```python
from build123d import *

# Parameters (mm, degrees)
SKETCH1_W           = 127
SKETCH1_H           = 127
BOSS_EXTRUDE1_DEPTH = 127
SKETCH2_W           = 96.52
SKETCH2_H           = 96.52
CUT_EXTRUDE1_DEPTH  = 118.11
SKETCH3_W           = 101.6
SKETCH3_H           = 101.6
SKETCH3_W_2         = 96.52
SKETCH3_H_2         = 96.52
CUT_EXTRUDE2_DEPTH  = 6.35
SKETCH5_W           = 96.52
SKETCH5_H           = 105.41
CUT_EXTRUDE3_DEPTH  = 6.35
SKETCH6_W           = 109.22
SKETCH6_H           = 105.41
CUT_EXTRUDE4_DEPTH  = 6.35
CHAMFER1_SIZE       = 1.016
FILLET2_R           = 0.762
FILLET3_R           = 0.762
FILLET4_R           = 0.762


with BuildPart() as part:
    # Sketch1 → Boss-Extrude1 (new body)
    with BuildSketch(Plane.XY):
        Rectangle(SKETCH1_W, SKETCH1_H)
    extrude(amount=BOSS_EXTRUDE1_DEPTH)

    # Sketch2 → Cut-Extrude1 (cut)
    with BuildSketch(Plane(origin=(0, 63.5, 0), x_dir=(1, 0, 0), z_dir=(0, 1, 0))):
        with Locations((0, -63.5)):
            Rectangle(SKETCH2_W, SKETCH2_H)
    extrude(amount=-CUT_EXTRUDE1_DEPTH, mode=Mode.SUBTRACT)

    # Sketch3 → Cut-Extrude2 (cut)
    with BuildSketch(Plane(origin=(0, 63.5, 0), x_dir=(1, 0, 0), z_dir=(0, 1, 0))):
        with Locations((0, -63.5)):
            Rectangle(SKETCH3_W, SKETCH3_H)
        with Locations((0, -63.5)):
            Rectangle(SKETCH3_W_2, SKETCH3_H_2, mode=Mode.SUBTRACT)
    extrude(amount=-CUT_EXTRUDE2_DEPTH, mode=Mode.SUBTRACT)

    # Sketch5 → Cut-Extrude3 (cut)
    with BuildSketch(Plane.XY.offset(15.24)):
        with Locations((0, -1.905)):
            Rectangle(SKETCH5_W, SKETCH5_H)
    cut_extrude3 = extrude(amount=-CUT_EXTRUDE3_DEPTH, mode=Mode.SUBTRACT)

    # Mirror1: Cut-Extrude3 across plane
    add(cut_extrude3.mirror(Plane(origin=(0, 0, 63.5), x_dir=(1, 0, 0), z_dir=(0, 0, -1))), mode=Mode.SUBTRACT)

    # Sketch6 → Cut-Extrude4 (cut)
    with BuildSketch(Plane.ZY.offset(-48.26)):
        with Locations((63.5, -1.905)):
            Rectangle(SKETCH6_W, SKETCH6_H)
    cut_extrude4 = extrude(amount=-CUT_EXTRUDE4_DEPTH, mode=Mode.SUBTRACT)

    # Mirror2: Cut-Extrude4 across plane
    add(cut_extrude4.mirror(Plane(origin=(0, 0, 0), x_dir=(0, 0, 1), z_dir=(1, 0, 0))), mode=Mode.SUBTRACT)

    # Chamfer1
    chamfer1_edges = [part.edges().sort_by_distance(p)[0] for p in [
        (0, -63.5, 127),
        (0, -63.5, 0),
        (63.5, -63.5, 63.5),
        (-63.5, -63.5, 63.5),
    ]]
    chamfer(chamfer1_edges, length=CHAMFER1_SIZE)

    # Fillet2
    fillet2_edges = [part.edges().sort_by_distance(p)[0] for p in [
        (54.61, -1.905, 8.89),
        (54.61, -1.905, 118.11),
        (-54.61, -1.905, 8.89),
        (-54.61, -1.905, 118.11),
    ]]
    fillet(fillet2_edges, radius=FILLET2_R)

    # Fillet3
    fillet3_edges = [part.edges().sort_by_distance(p)[0] for p in [
        (-50.8, 60.325, 114.3),
        (-50.8, 60.325, 12.7),
        (50.8, 60.325, 12.7),
        (50.8, 60.325, 114.3),
        (-48.26, 53.975, 15.24),
        (48.26, 53.975, 15.24),
        (48.26, 53.975, 111.76),
        (-48.26, 53.975, 111.76),
    ]]
    fillet(fillet3_edges, radius=FILLET3_R)

    # Fillet4
    fillet4_edges = [part.edges().sort_by_distance(p)[0] for p in [
        (54.61, 50.8, 63.5),
        (-54.61, 50.8, 63.5),
        (0, 50.8, 8.89),
        (0, 50.8, 118.11),
        (-54.386815367, 50.8, 9.113184633),
        (54.386815367, 50.8, 9.113184633),
        (-54.386815367, 50.8, 117.886815367),
        (54.386815367, 50.8, 117.886815367),
    ]]
    fillet(fillet4_edges, radius=FILLET4_R)


solid = part.part
```
Check sheet for the modelled part. Datum: model origin and axes. Units: mm. A direction names the side the tool comes from. Give positions to 0.01 mm unless a question says otherwise; leave off trailing zeros. Write each loop counter-clockwise with the first axis right and the second up, starting at its lowest first coordinate (ties: lowest second). Pieces come first, ordered by that corner, then holes.
Item 1: Gauge pin test, flat end, axial feed: pin 1 (8 mm diameter, centred on x = -23.5, z = 41, fed in from +Y). Record the tip position at first contact, or that the pin passes through.
Item 2: Cross-section at B-B (z = 63.5). Enter the section's corners in (x, y), and give its area (3 significant figures).
Item 3: Cross-section at D-D (y = -9). Enter the section's corners in (x, z).
Item 4: Draft check along X on faces 4 (the face through (-63.5, 0, 63)), 5 (the face through (0, 50.8, 11)), 6 (the face through (63.5, 0, 63)), 7 (the face through (-1, 54, 111.76)). Enter one of: released by +X, released by -X, zero draft, split by the parting line, or undercut.
Item 5: Cross-section at A-A (y = 54.5). Enter the section's corners in (x, z), and give its area (3 significant figures).
Item 6: Scan lines: L1, parallel to X at y = -23, z = 24; L2, parallel to Z at x = -27, y = 50; L3, parallel to X at y = 58, z = 35.5. Record each from-to range of solid material in increasing order.
Item 7: Cross-section at C-C (x = 18.5). Enter the section's corners in (y, z).
Item 8: Access from +Z, -Z, +X, -X, +Y, -Y to the whole of each face (thin tool, end or side, straight path). Record for faces 1 (the face through (-4, 57.15, 112)), 2 (the face through (-1, 1, 0)), 3 (the face through (-1, -2, 118.11)).
Report:
1. pin 1: stops at y = -54.61
2. outline: (-63.5, -62.48) - (-62.48, -63.5) - (62.48, -63.5) - (63.5, -62.48) - (63.5, 63.5) - (50.8, 63.5) - (50.8, 57.15) - (48.26, 57.15) - (48.26, 50.8) - (53.85, 50.8) arc R0.76 cw to (54.61, 50.04) - (54.61, -54.61) - (-54.61, -54.61) - (-54.61, 50.04) arc R0.76 cw to (-53.85, 50.8) - (-48.26, 50.8) - (-48.26, 57.15) - (-50.8, 57.15) - (-50.8, 63.5) - (-63.5, 63.5) - close
2. area: 3,360 mm2
3. outline: (-63.5, 0) - (63.5, 0) - (63.5, 127) - (-63.5, 127) - close; hole (-54.61, 9.65) arc R0.76 ccw to (-53.85, 8.89) - (53.85, 8.89) arc R0.76 ccw to (54.61, 9.65) - (54.61, 117.35) arc R0.76 ccw to (53.85, 118.11) - (-53.85, 118.11) arc R0.76 ccw to (-54.61, 117.35) - close
4. face 4: released by -X
4. face 5: undercut
4. face 6: released by +X
4. face 7: undercut
5. outline: (-63.5, 0) - (63.5, 0) - (63.5, 127) - (-63.5, 127) - close; hole (-48.26, 16) arc R0.76 ccw to (-47.5, 15.24) - (47.5, 15.24) arc R0.76 ccw to (48.26, 16) - (48.26, 111) arc R0.76 ccw to (47.5, 111.76) - (-47.5, 111.76) arc R0.76 ccw to (-48.26, 111) - close
5. area: 6,810 mm2
6. L1: x = -63.5 to -54.61, 54.61 to 63.5
6. L2: z = 0 to 8.89, 118.11 to 127
6. L3: x = -63.5 to -50.8, 50.8 to 63.5
7. outline: (-63.5, 1.02) - (-62.48, 0) - (63.5, 0) - (63.5, 12.7) - (57.15, 12.7) - (57.15, 15.24) - (50.8, 15.24) - (50.8, 9.65) arc R0.76 cw to (50.04, 8.89) - (-54.61, 8.89) - (-54.61, 118.11) - (50.04, 118.11) arc R0.76 cw to (50.8, 117.35) - (50.8, 111.76) - (57.15, 111.76) - (57.15, 114.3) - (63.5, 114.3) - (63.5, 127) - (-62.48, 127) - (-63.5, 125.98) - close
8. face 1: +Y
8. face 2: -Z, +X, -X, +Y, -Y
8. face 3: none
